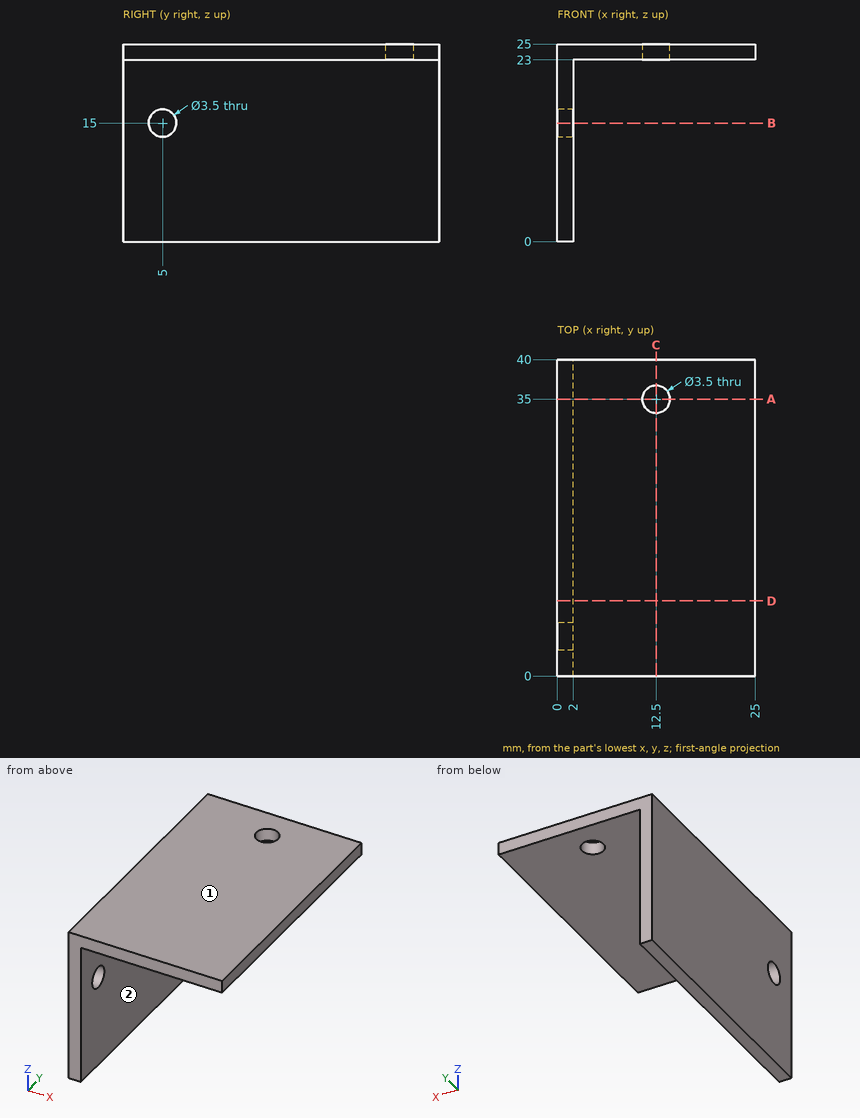
Can you work these out from the drawing? Everything is in mm from the part's minimum corner. A direction names the side the tool comes from. Coordinates: 2 decimals unless noted, no trailing zeros. Write each loop counter-clockwise with the first axis right and the second up, starting at its lowest first coordinate (ties: lowest second). Pieces come first, ordered by that corner, then holes. Notation, with made-up numbers: (74, 35.25) -> (117, 35.25) arc R14 cw to (117, 40.25) -> close; hole circle Ø8 at (66, 41). An arc over 180 degrees is marked (long way). Return JSON: item names as keys, results as strings.
(1) Imagine slicing it at B-B, the plane z = 15. Please give me the cut outline in (x, y).
Numbers:
{"outline": "(0, 0) -> (2, 0) -> (2, 3.25) -> (0, 3.25) -> close; (0, 6.75) -> (2, 6.75) -> (2, 40) -> (0, 40) -> close"}
(2) Imagine slicing it at C-C, the plane x = 12.5. Please give me the cut outline in (y, z), then the cut area to 3 significant figures.
Numbers:
{"outline": "(0, 23) -> (33.25, 23) -> (33.25, 25) -> (0, 25) -> close; (36.75, 23) -> (40, 23) -> (40, 25) -> (36.75, 25) -> close", "area": "73.0 mm2"}
(3) Which directions (+Z, -Z, +X, -X, +Y, -Y) give clear straight access to the entire face, cutting with the end or side of a thin tool? Please do the marked faces 1 and 2.
Numbers:
{"face 1": "+Z, +X, -X, +Y, -Y", "face 2": "-Z, +X, +Y, -Y"}
(4) I need wall thicknesses on L1, parallel to Z at x = 1.15, y = 5; L2, parallel to X at y = 35, z = 23.65; L3, parallel to Y at x = 0.7, z = 15. Which ranges of each line are inside material? Lowest first, please.
Numbers:
{"L1": "z = 0 to 13.25, 16.75 to 25", "L2": "x = 0 to 10.75, 14.25 to 25", "L3": "y = 0 to 3.25, 6.75 to 40"}
(5) Imagine slicing it at A-A, the plane y = 35. Please give me the cut outline in (x, z).
Numbers:
{"outline": "(0, 0) -> (2, 0) -> (2, 23) -> (10.75, 23) -> (10.75, 25) -> (0, 25) -> close; (14.25, 23) -> (25, 23) -> (25, 25) -> (14.25, 25) -> close"}
(6) Imagine slicing it at D-D, the plane y = 9.5. Please give me the cut outline in (x, z), then the cut area to 3 significant figures.
Numbers:
{"outline": "(0, 0) -> (2, 0) -> (2, 23) -> (25, 23) -> (25, 25) -> (0, 25) -> close", "area": "96.0 mm2"}
(7) I'm going to push flat-ended pins straight in: pin 1 (11.5 mm diameter, centred on x = 13, y = 10.5, fed in from -Z); pin 2 (3 mm diameter, centred on y = 18, z = 16.5, fed in from +X). Where does each tip first touch, or does it pass through?
Numbers:
{"pin 1": "stops at z = 23", "pin 2": "stops at x = 2"}
